Autodesk Inventor part; units mm, degrees
ref_plane "YZ Plane" through (0, 0, 0) normal (1, 0, 0) x (0, 1, 0)
ref_plane "XZ Plane" through (0, 0, 0) normal (0, 1, 0) x (-1, 0, 0)
ref_plane "XY Plane" through (0, 0, 0) normal (0, 0, 1) x (1, 0, 0)
sketch "スケッチ1" plane through (0, 0, 0) normal (0, 0, 1) x (1, 0, 0)
  circle A0 centre (0, 0) radius 10.5 construction
  circle A1 centre (-13.5, 1) radius 1.35
  line L0 (-13.5, 28) -> (13.5, 28) construction
  line L1 (13.5, 28) -> (13.5, 1) construction
  line L2 (13.5, 1) -> (-13.5, 1) construction
  line L3 (-13.5, 1) -> (-13.5, 28) construction
  circle A2 centre (-13.5, 28) radius 1.35
  circle A3 centre (13.5, 1) radius 1.35
  circle A4 centre (13.5, 28) radius 1.35
  line L4 (-19.75, 10) -> (-19.75, 7.1)
  line L5 (-19.75, 10) -> (19.75, 10)
  line L6 (19.75, 10) -> (19.75, 7.1)
  line L7 (-19.75, -7.1) -> (-19.75, -10)
  line L8 (-19.75, -10) -> (19.75, -10)
  line L9 (19.75, -7.1) -> (19.75, -10)
  line L10 (-19.75, 5) -> (-21.75, 5)
  line L11 (-21.75, 5) -> (-21.75, -5)
  line L12 (-21.75, -5) -> (-19.75, -5)
  arc A5 (-19.75, 5) -> (-19.75, 7.1) centre (-19.75, 6.05) ccw
  arc A6 (-19.75, -7.1) -> (-19.75, -5) centre (-19.75, -6.05) ccw
  line L13 (19.75, 5) -> (21.75, 5)
  line L14 (21.75, 5) -> (21.75, -5)
  line L15 (21.75, -5) -> (19.75, -5)
  arc A7 (19.75, 7.1) -> (19.75, 5) centre (19.75, 6.05) ccw
  line L16 (0, 28) -> (0, 0) construction
  arc A8 (19.75, -5) -> (19.75, -7.1) centre (19.75, -6.05) ccw
  line L17 (-21.75, 0) -> (21.75, 0) construction
  circle A9 centre (0, 0) radius 6.05
  point P0 (0, 10)
  dimension "d8" = 21
  dimension "d10" = 27
  dimension "d12" = 1
  dimension "d13" = 2.7
  dimension "d38" = 27
  dimension "d44" = 27
  dimension "d47" = 1.05
  dimension "d48" = 39.5
  dimension "d49" = 2
  dimension "d50" = 10
  dimension "d51" = 5
  dimension "d52" = 12.1
extrude "押し出し1" add sketch "スケッチ1" along normal blind 2 contours L5 L6 A7 L13 L14 L15 A8 L9 L8 L7 A6 L12 L11 L10 A5 L4
sketch "スケッチ2" plane through (0, 0, 2) normal (0, 0, 1) x (1, 0, 0)
  circle A0 centre (0, 0) radius 6.05
  circle A1 centre (13.5, 1) radius 1.35
  circle A2 centre (-13.5, 1) radius 1.35
  line L0 (-19.75, -10) -> (19.75, -10)
  line L1 (21.75, -5) -> (21.75, 5)
  line L2 (19.75, 10) -> (-19.75, 10)
  line L3 (21.75, 0) -> (0, 0) construction
  line L4 (13.5, -2) -> (7.7976, -2)
  arc A3 (-7.7976, -2) -> (7.7976, -2) centre (0, 0) ccw
  line L5 (-13.5, -2) -> (-7.7976, -2)
  line L6 (0, 0) -> (0, -6.05) construction
  circle A4 centre (0, 0) radius 6.05 construction
  arc A5 (13.5, 4) -> (10.6716, 2) centre (13.5, 1) ccw
  line L7 (10.6716, 2) -> (7.7976, 2)
  arc A6 (7.7976, 2) -> (-7.7976, 2) centre (0, 0) ccw
  line L8 (-7.7976, 2) -> (-10.6716, 2)
  arc A7 (-10.6716, 2) -> (-13.5, 4) centre (-13.5, 1) ccw
  line L9 (-13.5, 4) -> (-18.2897, 12.8425)
  line L10 (-18.2897, 12.8425) -> (18.2897, 12.8425)
  line L11 (18.2897, 12.8425) -> (13.5, 4)
  line L12 (-13.5, -2) -> (-18.8131, -15.0783)
  line L13 (-18.8131, -15.0783) -> (18.8131, -15.0783)
  line L14 (18.8131, -15.0783) -> (13.5, -2)
  line L15 (-16.75, 10) -> (-19.75, 10) construction
  line L16 (16.75, 10) -> (19.75, 10) construction
  line L17 (-19.75, -10) -> (19.75, -10) construction
  line L18 (-19.75, -10) -> (-16.75, -10) construction
  line L19 (16.75, -10) -> (19.75, -10) construction
  dimension "d55" = 2
  dimension "d56" = 2
  dimension "d57" = 3
  dimension "d61" = 3
  dimension "d62" = 3
extrude "押し出し2" cut sketch "スケッチ2" against normal blind 10 contours L12 L5 A3 L4 L14 L0 | L0 L14 L13 L12 | L11 A5 L7 A6 L8 A7 L9 L2
fillet "フィレット1" radius 2 14 edges at (7.7976, 2, 1) (7.7976, -2, 1) (-7.7976, -2, 1) (-7.7976, 2, 1) (13.5, -2, 1) (-13.5, -2, 1) (-13.5, 4, 1) (-10.6716, 2, 1) (10.6716, 2, 1) (13.5, 4, 1) (-16.75, 10, 1) (-16.75, -10, 1) (16.75, -10, 1) (16.75, 10, 1)
equation "\"d38\" = d10"
equation "\"d44\" = d10"
equation "\"d50\" = d11"
equation "\"d51\" = d12_1"
properties part number "足首_サブフレーム_1_2" material "アルミニウム 2014-T4"
Could you check a few things on this model? Use its own coordinates, in mm. A direction names the side the tool comes from. Give positions to 0.01 mm unless a question says otherwise; leave off trailing zeros. Loops run counter-clockwise (first coordinate to the right, second up) from the corner with the lowest first, then second, coordinate; pieces in that order, holes last. Notation, with made-up numbers: (-30.75, 57) - (-24.75, 57) arc R27 ccw to (-24.75, 96) - close; hole circle Ø10 at (3, 11). An arc over 180 degrees is marked (long way). Answer in a Markdown table with one row per item. Add a question column.
Q1. If we section it at A-A (y = -5.5): List the corners of the cut face in (x, z) for me, plus the area to 3 significant figures.
Q2. If we section it at B-B (x = -13.5): List the corners of the cut face in (y, z) for me.
Q3. If we section it at D-D (y = 1): List the corners of the cut face in (x, z) for me, plus the area to 3 significant figures.
Q4. For pin 1 (1 mm diameter, centred on x = 13, z = 0.5, fed in from -Y); pin 2 (0.6 mm diameter, centred on x = 20.5, z = 1, fed in from +Y); pin 3 (2.5 mm diameter, centred on x = -13.5, y = 1, fed in from +Z); pin 4 (1 mm diameter, centred on x = -11, z = 1, fed in from -Y), each with a flat end and sliding along its axis, tell me the tip position at first contact or that it passes through.
Q5. If we section it at C-C (z = 0.3): State how many separate pieces and enclosed holes the cut face has, plus the area to 3 significant figures.
Q6. We'd pull the mould along Y, two halves only. Please class faces 5 (the face through (5.589, 2.317, 0.986)), 6 (the face through (13.5, 4.3, 1)), 7 (the face through (-19.75, 9, 1)), 8 (the face through (18.7, -6.1, 1)): +Y half, -Y half, draft (parallel to the pull), parting line (faces both ways), or undercut.
Q7. Which directions (+Z, -Z, +X, -X, +Y, -Y) give clear straight access to the entire face, cutting with the end or side of a thin tool? Please do faces 1 (the face through (19, -10, 1)), 2 (the face through (-11.81, 3.48, 1.01)), 3 (the face through (21, 5, 1)), 4 (the face through (19.75, -9, 1)).
Q8. Please list where these lines run through material, in increasing order: L1, parallel to X at y = 7.25, z = 1.55; L2, parallel to X at y = -4.75, z = 0.1; L3, parallel to X at y = 5.5, z = 1.95. Write a range as from..to.
The answers:
| question | item | result |
|---|---|---|
| 1 | outline | (-18.86, 0) - (-14.92, 0) - (-14.92, 2) - (-18.86, 2) - close; (-5.88, 0) - (-2.52, 0) - (-2.52, 2) - (-5.88, 2) - close; (2.52, 0) - (5.88, 0) - (5.88, 2) - (2.52, 2) - close; (14.92, 0) - (18.86, 0) - (18.86, 2) - (14.92, 2) - close |
| 1 | area | 29.2 mm^2 |
| 2 | outline | (-2.52, 0) - (-0.35, 0) - (-0.35, 2) - (-2.52, 2) - close; (2.35, 0) - (4.3, 0) - (4.3, 2) - (2.35, 2) - close |
| 3 | outline | (-21.75, 0) - (-14.85, 0) - (-14.85, 2) - (-21.75, 2) - close; (-12.15, 0) - (-5.97, 0) - (-5.97, 2) - (-12.15, 2) - close; (5.97, 0) - (12.15, 0) - (12.15, 2) - (5.97, 2) - close; (14.85, 0) - (21.75, 0) - (21.75, 2) - (14.85, 2) - close |
| 3 | area | 52.3 mm^2 |
| 4 | pin 1 | stops at y = -2.52 |
| 4 | pin 2 | stops at y = 5 |
| 4 | pin 3 | passes through |
| 4 | pin 4 | stops at y = -2 |
| 5 | separate pieces | 1 |
| 5 | enclosed holes | 3 |
| 5 | area | 369 mm^2 |
| 6 | face 5 | undercut |
| 6 | face 6 | +Y half |
| 6 | face 7 | draft |
| 6 | face 8 | undercut |
| 7 | face 1 | +Z, -Z, +X, -X, -Y |
| 7 | face 2 | +Z, -Z, +Y |
| 7 | face 3 | +Z, -Z, +X, +Y |
| 7 | face 4 | +Z, -Z, +X, -Y |
| 8 | L1 | x = -19.75..-15.26, -3.5..3.5, 15.26..19.75 |
| 8 | L2 | x = -21.75..-14.62, -6.5..-3.75, 3.75..6.5, 14.62..21.75 |
| 8 | L3 | x = -18.86..-14.31, -5.88..-2.52, 2.52..5.88, 14.31..18.86 |
